Can you work these out from the model? Positions are in its coordinate system, mm. Give positions to 0.01 mm unless a question says otherwise; leave off trailing zeros. Loops run counter-clockwise (first coordinate to the right, second up) from the corner with the lowest first, then second, coordinate; pieces in that order, holes last. Notation, with made-up numbers: M 50,71.5 L 91,71.5 A30 ccw 91,109.5 Z; hole C -5.5,20.5 d3. An arc over 180 degrees is marked long. One line per item, written item: value. Start each with the question number.
Autodesk Inventor part; units mm, degrees
ref_plane "YZ Plane" through (0, 0, 0) normal (1, 0, 0) x (0, 1, 0)
ref_plane "XZ Plane" through (0, 0, 0) normal (0, 1, 0) x (-1, 0, 0)
ref_plane "XY Plane" through (0, 0, 0) normal (0, 0, 1) x (1, 0, 0)
sketch "Sketch1" plane through (0, 0, 0) normal (0, 0, 1) x (1, 0, 0)
  line L0 (-43.8671, 76.4402) -> (46.1329, 76.4402)
  line L1 (46.1329, 76.4402) -> (46.1329, -13.5598)
  line L2 (46.1329, -13.5598) -> (-43.8671, -13.5598)
  line L3 (-43.8671, -13.5598) -> (-43.8671, 76.4402)
  point P0 (0, 0)
  dimension "d0" = 90
  dimension "d1" = 90
extrude "Extrusion1" add sketch "Sketch1" along normal blind 6
sketch "Sketch2" plane through (0, 0, 0) normal (0, 0, -1) x (-1, 0, 0)
  line L0 (24.6671, 8.9402) -> (30.6671, 8.9402)
  line L1 (30.6671, 8.9402) -> (30.6671, 2.9402)
  line L2 (30.6671, 2.9402) -> (24.6671, 2.9402)
  line L3 (24.6671, 8.9402) -> (24.6671, 2.9402)
  line L4 (30.6671, 14.9402) -> (24.6671, 14.9402)
  line L5 (24.6671, 20.9402) -> (24.6671, 14.9402)
  line L6 (30.6671, 20.9402) -> (24.6671, 20.9402)
  line L7 (30.6671, 20.9402) -> (30.6671, 14.9402)
  line L8 (24.6671, 47.9402) -> (30.6671, 47.9402)
  line L9 (30.6671, 41.9402) -> (30.6671, 47.9402)
  line L10 (24.6671, 41.9402) -> (30.6671, 41.9402)
  line L11 (24.6671, 41.9402) -> (24.6671, 47.9402)
  line L12 (24.6671, 59.9402) -> (30.6671, 59.9402)
  line L13 (30.6671, 53.9402) -> (30.6671, 59.9402)
  line L14 (30.6671, 53.9402) -> (24.6671, 53.9402)
  line L15 (24.6671, 53.9402) -> (24.6671, 59.9402)
  line L16 (-32.9329, 47.9402) -> (-26.9329, 47.9402)
  line L17 (-26.9329, 41.9402) -> (-26.9329, 47.9402)
  line L18 (-32.9329, 41.9402) -> (-26.9329, 41.9402)
  line L19 (-32.9329, 41.9402) -> (-32.9329, 47.9402)
  line L20 (-32.9329, 59.9402) -> (-26.9329, 59.9402)
  line L21 (-26.9329, 53.9402) -> (-26.9329, 59.9402)
  line L22 (-26.9329, 53.9402) -> (-32.9329, 53.9402)
  line L23 (-32.9329, 53.9402) -> (-32.9329, 59.9402)
  line L24 (-26.9329, 14.9402) -> (-32.9329, 14.9402)
  line L25 (-32.9329, 20.9402) -> (-32.9329, 14.9402)
  line L26 (-26.9329, 20.9402) -> (-32.9329, 20.9402)
  line L27 (-26.9329, 20.9402) -> (-26.9329, 14.9402)
  line L28 (-32.9329, 8.9402) -> (-26.9329, 8.9402)
  line L29 (-26.9329, 8.9402) -> (-26.9329, 2.9402)
  line L30 (-26.9329, 2.9402) -> (-32.9329, 2.9402)
  line L31 (-32.9329, 8.9402) -> (-32.9329, 2.9402)
  line L32 (-32.9329, 8.9402) -> (-26.9329, 8.9402)
  line L33 (-26.9329, 8.9402) -> (-26.9329, 14.9402)
  line L34 (-26.9329, 14.9402) -> (-32.9329, 14.9402)
  line L35 (-32.9329, 14.9402) -> (-32.9329, 8.9402)
  line L36 (-32.9329, 2.9402) -> (-26.9329, 2.9402)
  line L37 (-26.9329, 2.9402) -> (-26.9329, -3.0598)
  line L38 (-26.9329, -3.0598) -> (-32.9329, -3.0598)
  line L39 (-32.9329, -3.0598) -> (-32.9329, 2.9402)
  line L40 (-32.9329, 47.9402) -> (-26.9329, 47.9402)
  line L41 (-26.9329, 47.9402) -> (-26.9329, 53.9402)
  line L42 (-26.9329, 53.9402) -> (-32.9329, 53.9402)
  line L43 (-32.9329, 53.9402) -> (-32.9329, 47.9402)
  line L44 (-32.9329, 59.9402) -> (-26.9329, 59.9402)
  line L45 (-26.9329, 59.9402) -> (-26.9329, 65.9402)
  line L46 (-26.9329, 65.9402) -> (-32.9329, 65.9402)
  line L47 (-32.9329, 65.9402) -> (-32.9329, 59.9402)
  line L48 (24.6671, 47.9402) -> (30.6671, 47.9402)
  line L49 (30.6671, 47.9402) -> (30.6671, 53.9402)
  line L50 (30.6671, 53.9402) -> (24.6671, 53.9402)
  line L51 (24.6671, 53.9402) -> (24.6671, 47.9402)
  line L52 (24.6671, 59.9402) -> (30.6671, 59.9402)
  line L53 (30.6671, 59.9402) -> (30.6671, 65.9402)
  line L54 (30.6671, 65.9402) -> (24.6671, 65.9402)
  line L55 (24.6671, 65.9402) -> (24.6671, 59.9402)
  line L56 (24.6671, 8.9402) -> (30.6671, 8.9402)
  line L57 (30.6671, 8.9402) -> (30.6671, 14.9402)
  line L58 (30.6671, 14.9402) -> (24.6671, 14.9402)
  line L59 (24.6671, 14.9402) -> (24.6671, 8.9402)
  line L60 (24.6671, 2.9402) -> (30.6671, 2.9402)
  line L61 (30.6671, 2.9402) -> (30.6671, -3.0598)
  line L62 (30.6671, -3.0598) -> (24.6671, -3.0598)
  line L63 (24.6671, -3.0598) -> (24.6671, 2.9402)
  point P0 (0, 0)
  dimension "d4" = 6
  dimension "d5" = 6
  dimension "d6" = 6
  dimension "d7" = 6
  dimension "d8" = 6
  dimension "d9" = 6
  dimension "d10" = 6
  dimension "d11" = 6
  dimension "d12" = 6
  dimension "d13" = 6
extrude "Extrusion2" cut sketch "Sketch2" against normal blind 6 contours L59 L4 L57 L0 | L2 L61 L62 L63 | L51 L14 L49 L8 | L55 L54 L53 L12 | L43 L22 L41 L16 | L47 L46 L45 L20 | L33 L28 L35 L24 | L37 L38 L39 L30
sketch "Sketch3" plane through (0, 0, 6) normal (0, 0, 1) x (1, 0, 0)
  circle A0 centre (-33.8671, -3.5598) radius 2
  line L0 (-43.8671, 76.4402) -> (-43.8671, -13.5598)
  line L1 (-43.8671, -13.5598) -> (46.1329, -13.5598)
  circle A1 centre (-33.8671, 6.4402) radius 2
  circle A2 centre (-33.8671, 16.4402) radius 2
  circle A3 centre (-33.8671, 26.4402) radius 2
  circle A4 centre (-33.8671, 36.4402) radius 2
  circle A5 centre (-33.8671, 46.4402) radius 2
  circle A6 centre (-33.8671, 56.4402) radius 2
  circle A7 centre (-33.8671, 66.4402) radius 2
  circle A8 centre (-23.8671, -3.5598) radius 2
  circle A9 centre (-23.8671, 6.4402) radius 2
  circle A10 centre (-23.8671, 16.4402) radius 2
  circle A11 centre (-23.8671, 26.4402) radius 2
  circle A12 centre (-23.8671, 36.4402) radius 2
  circle A13 centre (-23.8671, 46.4402) radius 2
  circle A14 centre (-23.8671, 56.4402) radius 2
  circle A15 centre (-23.8671, 66.4402) radius 2
  circle A16 centre (-13.8671, -3.5598) radius 2
  circle A17 centre (-13.8671, 6.4402) radius 2
  circle A18 centre (-13.8671, 16.4402) radius 2
  circle A19 centre (-13.8671, 26.4402) radius 2
  circle A20 centre (-13.8671, 36.4402) radius 2
  circle A21 centre (-13.8671, 46.4402) radius 2
  circle A22 centre (-13.8671, 56.4402) radius 2
  circle A23 centre (-13.8671, 66.4402) radius 2
  circle A24 centre (-3.8671, -3.5598) radius 2
  circle A25 centre (-3.8671, 6.4402) radius 2
  circle A26 centre (-3.8671, 16.4402) radius 2
  circle A27 centre (-3.8671, 26.4402) radius 2
  circle A28 centre (-3.8671, 36.4402) radius 2
  circle A29 centre (-3.8671, 46.4402) radius 2
  circle A30 centre (-3.8671, 56.4402) radius 2
  circle A31 centre (-3.8671, 66.4402) radius 2
  circle A32 centre (6.1329, -3.5598) radius 2
  circle A33 centre (6.1329, 6.4402) radius 2
  circle A34 centre (6.1329, 16.4402) radius 2
  circle A35 centre (6.1329, 26.4402) radius 2
  circle A36 centre (6.1329, 36.4402) radius 2
  circle A37 centre (6.1329, 46.4402) radius 2
  circle A38 centre (6.1329, 56.4402) radius 2
  circle A39 centre (6.1329, 66.4402) radius 2
  circle A40 centre (16.1329, -3.5598) radius 2
  circle A41 centre (16.1329, 6.4402) radius 2
  circle A42 centre (16.1329, 16.4402) radius 2
  circle A43 centre (16.1329, 26.4402) radius 2
  circle A44 centre (16.1329, 36.4402) radius 2
  circle A45 centre (16.1329, 46.4402) radius 2
  circle A46 centre (16.1329, 56.4402) radius 2
  circle A47 centre (16.1329, 66.4402) radius 2
  circle A48 centre (26.1329, -3.5598) radius 2
  circle A49 centre (26.1329, 6.4402) radius 2
  circle A50 centre (26.1329, 16.4402) radius 2
  circle A51 centre (26.1329, 26.4402) radius 2
  circle A52 centre (26.1329, 36.4402) radius 2
  circle A53 centre (26.1329, 46.4402) radius 2
  circle A54 centre (26.1329, 56.4402) radius 2
  circle A55 centre (26.1329, 66.4402) radius 2
  circle A56 centre (36.1329, -3.5598) radius 2
  circle A57 centre (36.1329, 6.4402) radius 2
  circle A58 centre (36.1329, 16.4402) radius 2
  circle A59 centre (36.1329, 26.4402) radius 2
  circle A60 centre (36.1329, 36.4402) radius 2
  circle A61 centre (36.1329, 46.4402) radius 2
  circle A62 centre (36.1329, 56.4402) radius 2
  circle A63 centre (36.1329, 66.4402) radius 2
  point P0 (0, 0)
  dimension "d16" = 4
  dimension "d18" = 10
  dimension "d21" = 10
  dimension "d24" = 10
  dimension "d27" = 10
extrude "Extrusion3" cut sketch "Sketch3" against normal blind 6 contours A0 | A1 | A2 | A3 | A4 | A5 | A6 | A7 | A16 | A17 | A18 | A19 | A20 | A21 | A22 | A23 | A24 | A25 | A26 | A27 | A28 | A29 | A30 | A31 | A32 | A33 | A34 | A35 | A36 | A37 | A38 | A39 | A40 | A41 | A42 | A43 | A44 | A45 | A46 | A47 | A56 | A57 | A58 | A59 | A60 | A61 | A62 | A63
sketch "Sketch4" plane through (0, 0, 0) normal (0, 0, -1) x (-1, 0, 0)
  line L0 (-32.9329, 20.9402) -> (-32.9329, 41.9402)
  line L1 (-32.9329, 20.9402) -> (-32.9329, 41.9402)
  line L2 (-32.9329, 41.9402) -> (-26.9329, 41.9402)
  line L3 (-32.9329, 41.9402) -> (-26.9329, 41.9402)
  line L4 (-32.9329, 41.9402) -> (-26.9329, 41.9402)
  line L5 (-32.9329, 20.9402) -> (-32.9329, 41.9402)
  line L6 (-26.9329, 41.9402) -> (-26.9329, 20.9402)
  line L7 (-26.9329, 20.9402) -> (-32.9329, 20.9402)
  point P0 (0, 0)
extrude "Extrusion4" cut sketch "Sketch4" against normal blind 6
sketch "Sketch5" plane through (0, 0, 6) normal (0, 0, 1) x (1, 0, 0)
  line L0 (-30.6671, 41.9402) -> (-30.6671, 20.9402)
  line L1 (-30.6671, 20.9402) -> (-24.6671, 20.9402)
  line L2 (-24.6671, 20.9402) -> (-24.6671, 41.9402)
  line L3 (-24.6671, 41.9402) -> (-30.6671, 41.9402)
  point P0 (0, 0)
extrude "Extrusion5" cut sketch "Sketch5" against normal blind 6
properties part number "FootScrewplate"
Q1. If we section it at B-B, the plane x = -4.5: Give the number of separate pieces and of enclosed holes in the cut face, plus the area to 3 significant figures.
Q2. If we mould it in two halves opening along Y, with no side actions, what happens to faces 1 (the face through (35.699, 34.488, 3.042)), 2 (the face through (-43.867, 31, 3))? For each: released by +Y, released by -Y, zero draft, split by the parting line, or undercut.
Q3. For P1, Ø3, axis at x = 16.13, y = 46.44, coming from the +Z side, with a flat end and sliding along its axis, tell me the tip position at first contact or that it passes through.
Q4. If we section it at A-A, the plane y = 12.5: Write out the boundary of the cut face in (x, z), plus the area to 3 significant figures.
Q5. I need wall thicknesses on line 1 along X through (y, z) = (64, 0.4); line 2 along Y through (x, z) = (29, 5.7). Which ranges of each line are inside material? Lowest first, please.
Response:
1. separate pieces: 9
1. enclosed holes: 0
1. area: 358 mm^2
2. face 1: undercut
2. face 2: zero draft
3. P1: through
4. outline: M -43.87,0 L -30.67,0 L -30.67,6 L -43.87,6 Z; M -24.67,0 L 26.93,0 L 26.93,6 L -24.67,6 Z; M 32.93,0 L 46.13,0 L 46.13,6 L 32.93,6 Z
4. area: 468 mm^2
5. line 1: -43.87 to -30.67, -24.67 to 26.93, 32.93 to 46.13
5. line 2: -13.56 to -3.06, 2.94 to 8.94, 14.94 to 20.94, 41.94 to 47.94, 53.94 to 59.94, 65.94 to 76.44
